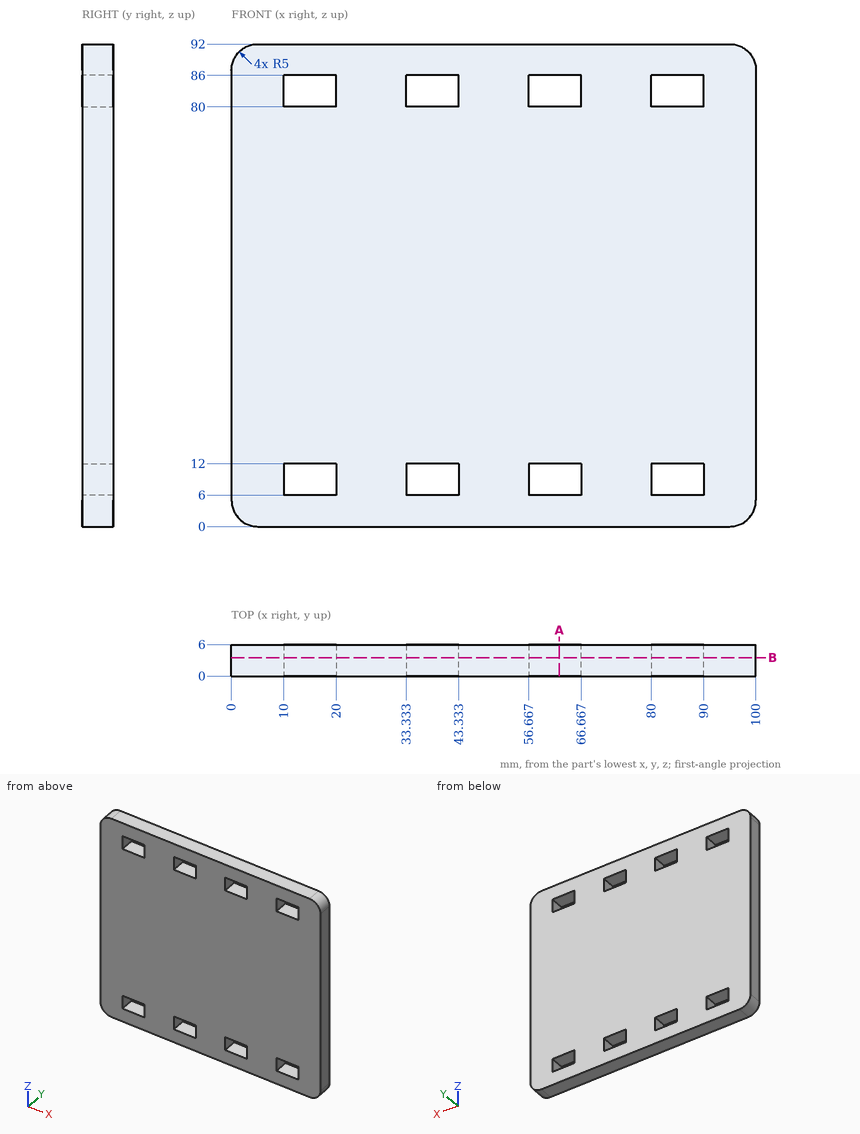
Geometry: see drawing. Coordinates: mm, zero at the bounding-box minimum. Round coordinates to 2 decimals unless told otherwise and drop trailing zeros. Order: outer loops, then holes, each group sorted by start corner. A loop starts at its lowest first (then second) coordinate and runs counter-clockwise, first axis right, second up. Notation, with made-up numbers: (87, 88.25) - (132, 88.25) arc R34 ccw to (132, 121.25) - close; hole circle Ø4 at (-38, 75.25). An arc over 180 degrees is marked (long way). One line per question, with ' | ' between items. Start each with the question number.
1) Cut plane B-B, the plane y = 3.5. Give the number of separate pieces and of enclosed holes in the cut face, then the cut area to 3 significant figures.
2) Ray query, probe 1 along X at (y, z) = (5, 84); probe 2 along Z at (x, y) = (37, 2.3); probe 3 along X at (y, z) = (2.7, 88.5). Return the intervals inside material, ascending.
3) Cut plane A-A, the plane x = 62.5. Return the cut outline in (y, z).
Worked out:
1) separate pieces: 1 | enclosed holes: 8 | area: 8,700 mm^2
2) probe 1: x = 0 to 10, 20 to 33.33, 43.33 to 56.67, 66.67 to 80, 90 to 100 | probe 2: z = 0 to 6, 12 to 80, 86 to 92 | probe 3: x = 0.23 to 99.77
3) outline: (0, 0) - (6, 0) - (6, 6) - (0, 6) - close; (0, 12) - (6, 12) - (6, 80) - (0, 80) - close; (0, 86) - (6, 86) - (6, 92) - (0, 92) - close
